Part model, mm, in its own coordinate system. A direction names the side the tool comes from. Coordinates: 2 decimals unless noted, no trailing zeros. Write each loop counter-clockwise with the first axis right and the second up, starting at its lowest first coordinate (ties: lowest second). Pieces come first, ordered by that corner, then holes. Notation, with made-up numbers: (53, 89) - (60, 89) arc R20 ccw to (60, 122) - close; hole circle Ø2 at (79.5, 3). An arc over 180 degrees is marked (long way). Write each question's results on one line, items separated by ' | '.
Autodesk Inventor part; units mm, degrees
ref_plane "YZ Plane" through (0, 0, 0) normal (1, 0, 0) x (0, 1, 0)
ref_plane "XZ Plane" through (0, 0, 0) normal (0, 1, 0) x (-1, 0, 0)
ref_plane "XY Plane" through (0, 0, 0) normal (0, 0, 1) x (1, 0, 0)
sketch "Sketch1" plane through (0, 0, 0) normal (0, 0, 1) x (1, 0, 0)
  circle A0 centre (0, 0) radius 1.5
  line L0 (2.5, 2.5) -> (-4, 2.5)
  line L1 (-4, 2.5) -> (-4, -2.5)
  line L2 (-4, -2.5) -> (2.5, -2.5)
  line L3 (2.5, -2.5) -> (2.5, 2.5)
  dimension "d0" = 3
  dimension "d1" = 1
  dimension "d2" = 1
  dimension "d3" = 1
  dimension "d4" = 2.5
extrude "Extrusion1" add sketch "Sketch1" along normal blind 2
sketch "Sketch2" plane through (-4, -2.5, 0) normal (-1, 0, 0) x (0, 0, 1)
  line L0 (0, 0) -> (2, 0)
  line L1 (0, 0) -> (6.5, 0)
  line L2 (6.5, 0) -> (6.5, 5)
  line L3 (6.5, 5) -> (0, 5)
  line L4 (0, 5) -> (0, 0)
  circle A0 centre (4, 2.5) radius 1.5
  point P0 (0, 2.5)
  dimension "d7" = 3
  dimension "d8" = 2.5
  dimension "d9" = 1
  dimension "d10" = 1
  dimension "d11" = 1
extrude "Extrusion2" add sketch "Sketch2" against normal blind 2
fillet "Fillet2" radius 0.5 1 edges at (-2, 0, 2)
fillet "Fillet2" radius 1 6 edges at (0.25, 2.5, 2) (-2, 2.5, 4.25) (-2, 0, 6.5) (-2, -2.5, 4.25) (0.25, -2.5, 2) (2.5, 0, 2)
properties part number "draat tap stukje 1"
(1) 3-axis set-ups, long thin cutter, end or side, ignore diameter. For faces 1 (the cylindrical face through (-2.301, -2.215, 4.528)), 2 (the cylindrical face through (-2.301, 2.215, 4.472)), 3 (the cylindrical face through (-1.5, -0.07, 0.99)): which of +Z, -Z, +X, -X, +Y, -Y reach the whole face in a straight line?
Return value:
face 1: +Z, +X, -Y | face 2: +Z, +X, +Y | face 3: +Z, -Z
(2) Saw through at C-C on y = 0. Count the separate pieces of the cut face and the enclosed holes in it, then the cut area to 3 significant figures.
Return value:
separate pieces: 3 | enclosed holes: 0 | area: 9.62 mm^2
(3) Two-plate mould, pull along Y, no slides. Class faces 4 (the flat face through (-2.4, 2.5, 1.1)), 5 (the cylindrical face through (-3.014, -0.575, 5.386)), 6 (the flat face through (-3.5, 0, 6.5)): released by +Y, released by -Y, zero draft, split by the parting line, or undercut.
Return value:
face 4: released by +Y | face 5: undercut | face 6: zero draft
(4) Flat gauge pins, fed straight in: P1, Ø2.5, axis at x = -0.5, y = 0.5, coming from the +Z side; P2, Ø3, axis at x = 1, y = -2, coming from the +Z side. Where does each tip first touch, or does it go through?
Return value:
P1: stops at z = 2.07 | P2: stops at z = 2
(5) Saw through at D-D on x = -3.5. Write the cut outline in (y, z).
Return value:
outline: (-2.5, 0) - (2.5, 0) - (2.5, 6.5) - (-2.5, 6.5) - close; hole circle Ø3 at (0, 4)
(6) Wall check: line 1 (Z direction, x = 1.25, y = 1.3); line 2 (Y direction, x = -0.5, z = 1); line 3 (X direction, y = -0.4, z = 1.5). Give the ranges that are in metal, low to high. Write a range as from..to.
Return value:
line 1: z = 0..2 | line 2: y = -2.5..-1.41, 1.41..2.5 | line 3: x = -4..-1.45, 1.45..2.37
